Design review of the part built by this model. Coordinates are the model's own, in mm. Round coordinates to 2 decimals unless told otherwise and drop trailing zeros. Write each loop counter-clockwise with the first axis right and the second up, starting at its lowest first coordinate (ties: lowest second). Pieces come first, ordered by that corner, then holes. Notation, with made-up numbers: M -29,71.25 L 19,71.25 A30 cw 19,94.25 Z; hole C -24,-14 d9. An arc over 180 degrees is marked long. One line per question, with ' | ' between items. Start each with the question number.
Item 1: Add section C-C, the plane x = -0.5. State the section outline as (y, z) points.
Item 2: Add section A-A, the plane z = -29. State the section outline as (x, y) points.
Item 3: Add section D-D, the plane y = 8.5. State the section outline as (x, z) points, and give its area (3 significant figures).
Item 4: For L1, parallel to Z at x = 3, y = 15; L2, parallel to X at y = 8.25, z = -29; L3, parallel to Y at x = 1.5, z = -28.5, list the stretches that pass through material, from the lowest coordinate up.
Item 5: Draft analysis for pull direction Z (two halves, no side actions). For faces 1 (the face through (4, 8, -35)), 2 (the face through (-2, 4, -2)), 3 (the face through (2.22, 15.81, -31.55)), state which applies: released by +Z, released by -Z, zero draft, split by the parting line, or undercut.
Item 6: Insertion check: pin 1 Ø5 at (y, z) = (5, -8.5) entering from -X; pin 2 Ø4 at (x, y) = (-1, 5) entering from -Z; pin 3 Ø1 at (x, y) = (-1, 18) entering from -Z. Each pin has a flat end and moves straight along its axis. Give the tip position at first contact, or say it passes through.
Item 7: Add section B-B, the plane y = 11.25. State the section outline as (x, z) points, and give its area (3 significant figures).
```python
from build123d import *

# Parameters (mm, degrees)
SKETCH037_R     = 1.75
PAD011_DEPTH    = 4.5
PAD012_DEPTH    = 4.5
POCKET012_DEPTH = 9
CHAMFER006_SIZE = 1


with BuildPart() as body017:
    # Sketch037 → Pad011 (new body)
    with BuildSketch(Plane.YZ):
        with BuildLine():
            ThreePointArc((4.76184, 4.428443), (2.507235, 5.596958), (0, 6))
            Line((0, -35.5), (0, 6))
            Line((15.000002, -35.5), (0, -35.5))
            ThreePointArc((15.000002, -35.5), (18.889094, -33.88908), (20.5, -29.999981))
            Line((20.5, -10.000019), (20.5, -29.999981))
            ThreePointArc((20.5, -10.000019), (19.912019, -7.525718), (18.273777, -5.580455))
            Line((18.273777, -5.580455), (4.76184, 4.428443))
        make_face()
        with Locations((15, -10)):
            Circle(SKETCH037_R, mode=Mode.SUBTRACT)
        with Locations((15, -30)):
            Circle(SKETCH037_R, mode=Mode.SUBTRACT)
    extrude(amount=-PAD011_DEPTH)

    # Sketch038 (on Pad) → Pad012 (join)
    with BuildSketch(Plane.YZ):
        with BuildLine():
            ThreePointArc((0, -6), (4, -2), (0, 2))
            Line((0, 2), (0, -6))
        make_face()
    extrude(amount=PAD012_DEPTH)

    # Sketch039 (on Face5 of Pad012) → Pocket012 (cut)
    with BuildSketch(Plane(origin=(-4.5, 0, 0), x_dir=(0, 1, 0), z_dir=(-1, 0, 0))):
        with BuildLine():
            ThreePointArc((0, 0.8), (1.2, 2), (0, 3.2))
            Line((0, 3.2), (0, 0.8))
        make_face()
    extrude(amount=-POCKET012_DEPTH, mode=Mode.SUBTRACT)

    # Chamfer006
    chamfer006_edges = [body017.edges().sort_by_distance(p)[0] for p in [
        (-4.5, 7.500001, -35.5),
    ]]
    chamfer(chamfer006_edges, length=CHAMFER006_SIZE)


with BuildPart() as part_mirroring011:
    # Part__Mirroring011: instance of Body017
    add(body017.part.mirror(Plane(origin=(0, 0, 0), x_dir=(0, -1, 0), z_dir=(1, 0, 0))))


solid = part_mirroring011.part
```
Computed values:
1) outline: M 0,-6 A4 ccw 0,2 L 0,-0.8 A1.2 cw 0,-3.2 Z
2) outline: M 0,0 L 4.5,0 L 4.5,13.56 L 0,13.56 Z; M 0,16.44 L 4.5,16.44 L 4.5,19.5 L 3.5,20.5 L 0,20.5 Z
3) outline: M 0,-35.5 L 3.5,-35.5 L 4.5,-34.5 L 4.5,0.41 L 3.5,1.66 L 0,1.66 Z | area: 166 mm^2
4) L1: z = -35.5 to -31.75, -28.25 to -11.75, -8.25 to -3.16 | L2: x = 0 to 4.5 | L3: y = 0 to 14.1, 15.9 to 20.5
5) face 1: released by -Z | face 2: split by the parting line | face 3: undercut
6) pin 1: stops at x = 0 | pin 2: stops at z = -35.5 | pin 3: passes through
7) outline: M 0,-35.5 L 3.5,-35.5 L 4.5,-34.5 L 4.5,-1.62 L 3.5,-0.38 L 0,-0.38 Z | area: 157 mm^2
